```python
from build123d import *

# Parameters (mm, degrees)
PAD_DEPTH    = 5
PAD001_DEPTH = 5
PAD002_DEPTH = 10


with BuildPart() as part:
    # Sketch → Pad (new body, symmetric)
    with BuildSketch(Plane.YZ):
        with BuildLine():
            Line((79.985253, 20.323011), (100.763572, 40.6142))
            Line((100.763572, 40.6142), (119.662178, 40.6142))
            Line((119.662178, 40.6142), (119.662178, 18.903042))
            Line((119.662178, 18.903042), (100.307594, -20.290001))
            Line((100.307594, -20.290001), (-84.034331, -20.290001))
            ThreePointArc((-85.010115, 20.323011), (-105.527296, -0.488171), (-84.034331, -20.290001))
            Line((-85.010115, 20.323011), (-29.368151, 20.323011))
            ThreePointArc((29.663353, 20.323011), (0.147601, 49.838763), (-29.368151, 20.323011))
            Line((29.663353, 20.323011), (79.985253, 20.323011))
        make_face()
    extrude(amount=PAD_DEPTH, both=True)

    # Sketch001 → Pad001 (join, symmetric)
    with BuildSketch(Plane.XY):
        Polygon((-82.730919, -11.478452), (-82.730919, 53.577414), (0, 5.912332), (82.730919, 53.577414), (82.730919, -11.478452), (0, -78.832466), align=None)
    extrude(amount=PAD001_DEPTH, both=True)

    # Sketch002 (on Face1 of Pad001) → Pad002 (join)
    with BuildSketch(Plane(origin=(0, 0, 20.323011), x_dir=(0, -1, 0), z_dir=(0, 0, 1))):
        Polygon((-77.402542, 41.444447), (-77.402542, -41.444447), (-36.757927, -19.18667), (-36.757927, 19.18667), align=None)
    extrude(amount=-PAD002_DEPTH)


solid = part.part
```
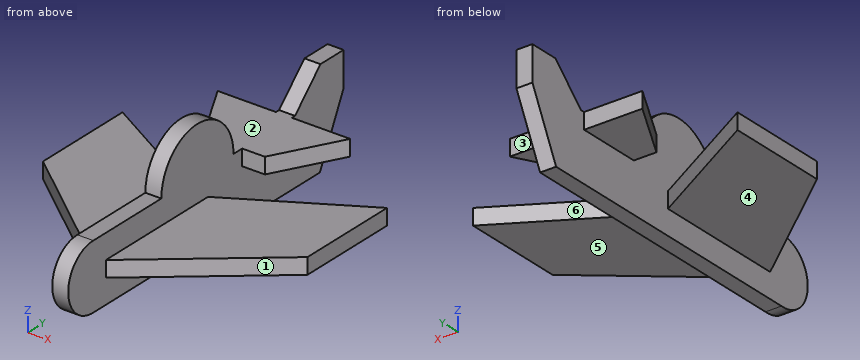
CAD build for the part. Positions are in the model's coordinates, mm. Face numbers are marked on the shaded views. A direction names the side the tool comes from. Round coordinates to 2 decimals unless told otherwise and drop trailing zeros. Order: outer loops, then holes, each group sorted by start corner. A loop starts at its lowest first (then second) coordinate and runs counter-clockwise, first axis right, second up. Notation, with made-up numbers: (89, -21.75) -> (132, -21.75) arc R32 ccw to (132, 15.25) -> close; hole circle Ø6 at (45, 29). An arc over 180 degrees is marked (long way). One line per question, with ' | ' between items.
Q1. Which spindle directions (+Z, -Z, +X, -X, +Y, -Y) get a long thin tool onto all of the face, cutting with end or side? Do the marked faces 4, 5 and 6. Say none if no direction does.
Completed:
face 4: -Z, -X, +Y, -Y | face 5: -Z, +X, +Y, -Y | face 6: +Z, -Z, +Y
Q2. Slice it at C-C (y = -33.5). Write the cut outline in (x, z), then the cut area to 3 significant figures.
Completed:
outline: (-55.68, -5) -> (-5, -5) -> (-5, -20.29) -> (5, -20.29) -> (5, -5) -> (55.68, -5) -> (55.68, 5) -> (5, 5) -> (5, 20.32) -> (-5, 20.32) -> (-5, 5) -> (-55.68, 5) -> close | area: 1,420 mm^2
Q3. Probe probe 1 along X at (y, z) = (37.5, 2); probe 2 along X at (y, z) = (16, -7); probe 3 along Z at (x, y) = (-2, -60.5). List the from-to ranges inside material, lowest first.
Completed:
probe 1: x = -82.73 to -54.83, -5 to 5, 54.83 to 82.73 | probe 2: x = -5 to 5 | probe 3: z = -20.29 to 20.32
Q4. Two-plate mould, pull along Y, no slides. Class the marked faces 1, 2 and 3: released by +Y, released by -Y, zero draft, split by the parting line, or undercut.
Completed:
face 1: released by -Y | face 2: undercut | face 3: released by +Y
Q5. Drop flat-ended pins along their axis: pin 1 (11 mm diameter, centred on x = -11.5, z = 16, fed in from -Y); pin 2 (11 mm diameter, centred on x = 2, y = 113.5, fed in from +Z); pin 3 (1.5 mm diameter, centred on y = -46.5, z = 12, fed in from +X); pin 4 (6 mm diameter, centred on x = -33.5, z = -9.5, fed in from +Y). Give the stop position or say it passes through.
Completed:
pin 1: stops at y = 36.76 | pin 2: stops at z = 40.61 | pin 3: stops at x = 5 | pin 4: passes through
Q6. Slice it at D-D (z = 0). Write the cut outline in (x, y), then the cut area to 3 significant figures.
Completed:
outline: (-82.73, -11.48) -> (-5, -74.76) -> (-5, -105.53) -> (5, -105.53) -> (5, -74.76) -> (82.73, -11.48) -> (82.73, 53.58) -> (5, 8.79) -> (5, 110.33) -> (-5, 110.33) -> (-5, 8.79) -> (-82.73, 53.58) -> close | area: 13,700 mm^2
Q7. Slice it at B-B (x = -30.5). Write the cut outline in (y, z).
Completed:
outline: (-54, -5) -> (23.48, -5) -> (23.48, 5) -> (-54, 5) -> close; (57.42, 10.32) -> (77.4, 10.32) -> (77.4, 20.32) -> (57.42, 20.32) -> close
Q8. Slice it at A-A (z = 26.5). Write the cut outline in (x, y).
Completed:
outline: (-5, -28.71) -> (5, -28.71) -> (5, 29.01) -> (-5, 29.01) -> close; (-5, 86.31) -> (5, 86.31) -> (5, 119.66) -> (-5, 119.66) -> close
